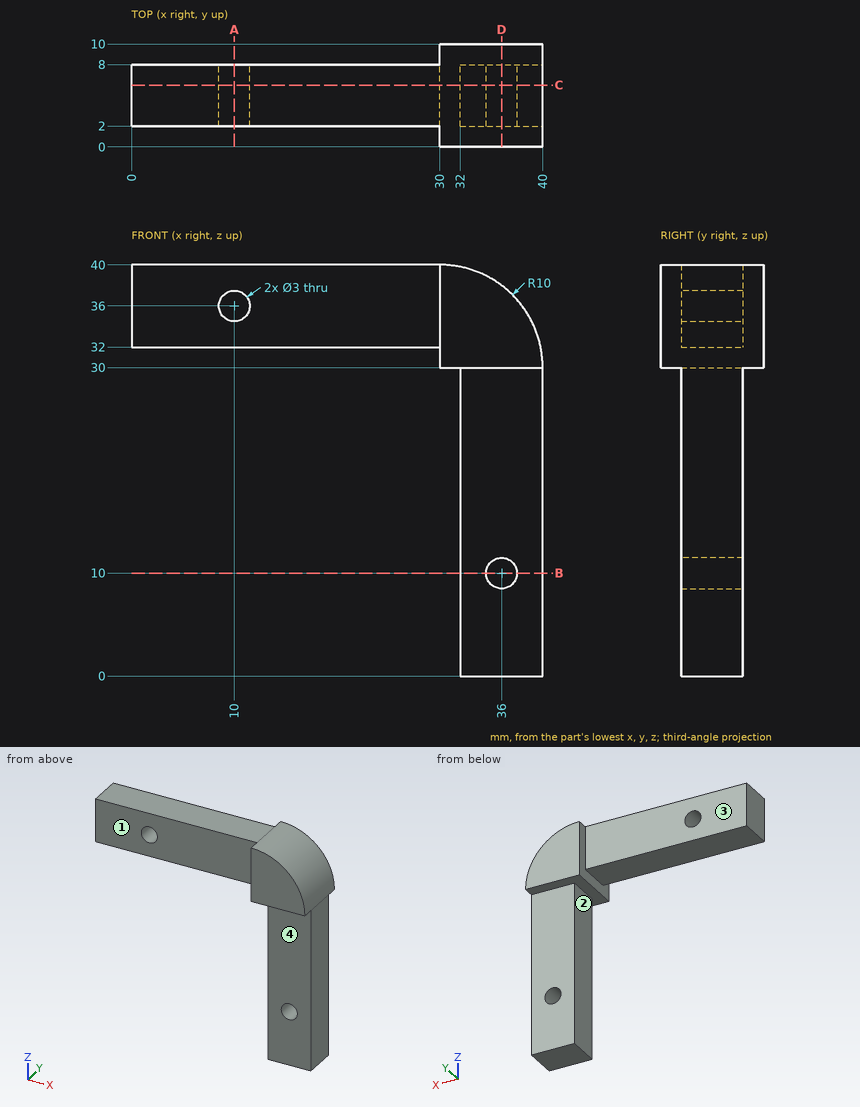
Verification items for this drawing (mm, ordinates from the low corner). A direction names the side the tool comes from. Give positions to 0.01 mm unless a question says otherwise; leave off trailing zeros. Order: outer loops, then holes, each group sorted by start corner. A loop starts at its lowest first (then second) coordinate and runs counter-clockwise, first axis right, second up.
1) Gauge pin test, flat ends, axial feed: pin 1 (10 mm diameter, centred on x = 35, z = 24, fed in from +Y); pin 2 (4 mm diameter, centred on x = 37, z = 9.5, fed in from -Y); pin 3 (2 mm diameter, centred on y = 2.5, z = 31.5, fed in from -X); pin 4 (2.5 mm diameter, centred on x = 10, z = 36, fed in from +Y). Record the tip position at first contact, or that the pin passes through.
Results are:
pin 1: stops at y = 8
pin 2: stops at y = 2
pin 3: stops at x = 0
pin 4: passes through
2) Cross-section at D-D (x = 36). Record the boundary of the cut face in (y, z), then the cut area to 3 significant figures.
Results are:
outline: (0, 30) - (2, 30) - (2, 11.5) - (8, 11.5) - (8, 30) - (10, 30) - (10, 38) - (0, 38) - close; (2, 0) - (8, 0) - (8, 8.5) - (2, 8.5) - close
area: 242 mm2
3) Material ranges on probe 1 along X at (y, z) = (4.8, 10); probe 2 along Y at (x, z) = (28.5, 38.5); probe 3 along X at (y, z) = (6.5, 11), recorded low to high.
Results are:
probe 1: x = 32 to 34.5, 37.5 to 40
probe 2: y = 2 to 8
probe 3: x = 32 to 34.88, 37.12 to 40
4) Cross-section at A-A (x = 10). Record the boundary of the cut face in (y, z), then the cut area to 3 significant figures.
Results are:
outline: (2, 32) - (8, 32) - (8, 34.5) - (2, 34.5) - close; (2, 37.5) - (8, 37.5) - (8, 40) - (2, 40) - close
area: 30.0 mm2
5) Tool access check on the marked faces 1, 2, 3 and 4. Record the directions out of +Z, -Z, +X, -X, +Y, -Y that give a thin tool (end or side, any length) a straight path to the whole face; none if there is none.
Results are:
face 1: +Z, -Z, -X, -Y
face 2: -Z, -X, +Y, -Y
face 3: +Z, -Z, -X, +Y
face 4: -Z, +X, -X, -Y
6) Cross-section at C-C (y = 6). Record the boundary of the cut face in (x, z).
Results are:
outline: (0, 32) - (30, 32) - (30, 30) - (32, 30) - (32, 0) - (40, 0) - (40, 30) arc R10 ccw to (30, 40) - (0, 40) - close; hole circle Ø3 at (10, 36); hole circle Ø3 at (36, 10)
7) Cross-section at B-B (z = 10). Record the boundary of the cut face in (x, y), then the cut area to 3 significant figures.
Results are:
outline: (32, 2) - (34.5, 2) - (34.5, 8) - (32, 8) - close; (37.5, 2) - (40, 2) - (40, 8) - (37.5, 8) - close
area: 30.0 mm2
